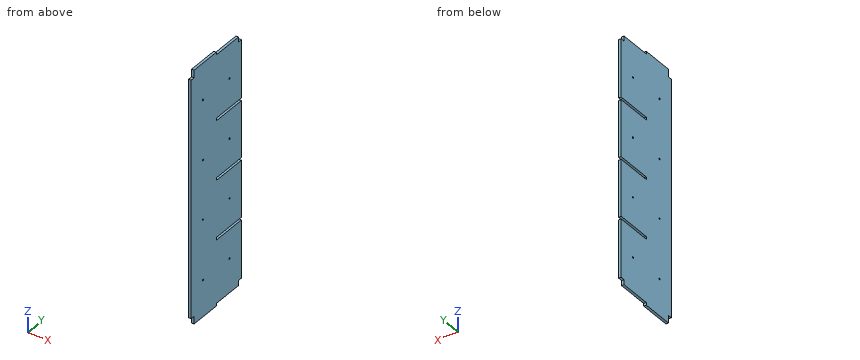
```python
from build123d import *

# Parameters (mm, degrees)
BOSS_EXTRUDE1_DEPTH = 6
SKETCH2_W           = 6.2
SKETCH2_H           = 85
CUT_EXTRUDE1_DEPTH  = 6
SKETCH3_R           = 2
CUT_EXTRUDE2_DEPTH  = 6


with BuildPart() as part:
    # Sketch1 → Boss-Extrude1 (new body)
    with BuildSketch(Plane(origin=(0, 0, 0), x_dir=(0, 0, -1), z_dir=(1, 0, 0))):
        Polygon((0, 0), (560, 0), (560, 10), (578, 10), (578, 85), (571.9, 85), (571.9, 160), (560, 160), (560, 170), (0, 170), (0, 160), (-11.9, 160), (-11.9, 85), (-18, 85), (-18, 10), (0, 10), align=None)
    extrude(amount=BOSS_EXTRUDE1_DEPTH)

    # Sketch2 → Cut-Extrude1 (cut)
    with BuildSketch(Plane(origin=(6, 0, 0), x_dir=(0, 0, -1), z_dir=(1, 0, 0))):
        with Locations((140, 127.5)):
            Rectangle(SKETCH2_W, SKETCH2_H)
        with Locations((280, 127.5)):
            Rectangle(SKETCH2_W, SKETCH2_H)
        with Locations((420, 127.5)):
            Rectangle(SKETCH2_W, SKETCH2_H)
    extrude(amount=-CUT_EXTRUDE1_DEPTH, mode=Mode.SUBTRACT)

    # Sketch3 → Cut-Extrude2 (cut)
    with BuildSketch(Plane(origin=(6, 0, 0), x_dir=(0, 0, -1), z_dir=(1, 0, 0))):
        with Locations((68.45, 130)):
            Circle(SKETCH3_R)
        with Locations((68.45, 40)):
            Circle(SKETCH3_R)
        with Locations((210, 130)):
            Circle(SKETCH3_R)
        with Locations((210, 40)):
            Circle(SKETCH3_R)
        with Locations((350, 130)):
            Circle(SKETCH3_R)
        with Locations((350, 40)):
            Circle(SKETCH3_R)
        with Locations((491.55, 130)):
            Circle(SKETCH3_R)
        with Locations((491.55, 40)):
            Circle(SKETCH3_R)
    extrude(amount=-CUT_EXTRUDE2_DEPTH, mode=Mode.SUBTRACT)


solid = part.part
```
Design review of the part built by this model. Coordinates are the model's own, in mm. Round coordinates to 2 decimals unless told otherwise and drop trailing zeros. Write each loop counter-clockwise with the first axis right and the second up, starting at its lowest first coordinate (ties: lowest second). Pieces come first, ordered by that corner, then holes. Notation, with made-up numbers: (-16.5, 29) -> (1.5, 29) arc R21 cw to (1.5, 65) -> close; hole circle Ø11 at (32.5, 61.25). An arc over 180 degrees is marked (long way). Answer in a Markdown table with one row per item.
Q1. Take a section at A-A, the plane y = 151.5. State the section outline as (x, z) points.
The answers:
| item | result |
|---|---|
| outline | (0, -571.9) -> (6, -571.9) -> (6, -423.1) -> (0, -423.1) -> close; (0, -416.9) -> (6, -416.9) -> (6, -283.1) -> (0, -283.1) -> close; (0, -276.9) -> (6, -276.9) -> (6, -143.1) -> (0, -143.1) -> close; (0, -136.9) -> (6, -136.9) -> (6, 11.9) -> (0, 11.9) -> close |
Q2. To check wall thickness, follow L1, parallel to Z at x = 0.4, y = 150.5; L2, parallel to Y at x = 1.45, z = -68.45; L3, parallel to Y at x = 1.6, z = -351. State the ranges of each line that lie inside material, in increasing order. Write a range as [from, to].
The answers:
| item | result |
|---|---|
| L1 | [-571.9, -423.1], [-416.9, -283.1], [-276.9, -143.1], [-136.9, 11.9] |
| L2 | [0, 38], [42, 128], [132, 170] |
| L3 | [0, 38.27], [41.73, 128.27], [131.73, 170] |
Q3. Take a section at B-B, the plane x = 2.3. Count the separate pieces of the cut face and the enclosed holes in it, then the cut area to 3 significant figures.
The answers:
| item | result |
|---|---|
| separate pieces | 1 |
| enclosed holes | 8 |
| area | 98,000 mm² |
Q4. Clearance check with flat-ended pins moving along their axes: pin 1 Ø2.5 at (y, z) = (130, -68.45) entering from -X; pin 2 Ø12 at (y, z) = (125.5, -282.5) entering from -X; pin 3 Ø3 at (x, z) = (1.5, -140) entering from +Y; pin 4 Ø3 at (x, y) = (2.5, 166.5) entering from -Z. State where each tip first meets the part, or that it passes through.
The answers:
| item | result |
|---|---|
| pin 1 | through |
| pin 2 | x = 0 |
| pin 3 | y = 85 |
| pin 4 | z = -560 |
